Autodesk Inventor part; units mm, degrees
ref_plane "YZ Plane" through (0, 0, 0) normal (1, 0, 0) x (0, 1, 0)
ref_plane "XZ Plane" through (0, 0, 0) normal (0, 1, 0) x (-1, 0, 0)
ref_plane "XY Plane" through (0, 0, 0) normal (0, 0, 1) x (1, 0, 0)
sketch "Schizzo1" plane through (0, 0, 0) normal (0, 1, 0) x (-1, 0, 0)
  circle A0 centre (0, 0) radius 3.25
  circle A1 centre (0, 0) radius 6.5
  dimension "d0" = 6.5
  dimension "d1" = 13
extrude "Estrusione1" add sketch "Schizzo1" along normal blind 15
sketch "Schizzo2" plane through (0, 0, 0) normal (0, -1, 0) x (1, 0, 0)
  line L0 (-13.5, -10) -> (13.5, -10)
  line L1 (13.5, -10) -> (13.5, 10)
  line L2 (13.5, 10) -> (-13.5, 10)
  line L3 (-13.5, 10) -> (-13.5, -10)
  line L4 (-13.5, -10) -> (13.5, 10) construction
  line L5 (13.5, -10) -> (-13.5, 10) construction
  point P0 (0, 0)
  point P1 (0, 0)
  point P2 (0, 0)
  dimension "d4" = 20
  dimension "d5" = 27
extrude "Estrusione2" add sketch "Schizzo2" along normal blind 3
sketch "Schizzo3" plane through (0, -3, 0) normal (0, -1, 0) x (1, 0, 0)
  line L0 (0, 0) -> (-8, 0)
  line L1 (0, 0) -> (8, 0) construction
  line L2 (-8, 0) -> (-8, -5.5)
  line L3 (0, 0) -> (8, 0)
  line L4 (0, 0) -> (8, 0) construction
  line L5 (8, 0) -> (8, -5.5)
  circle A0 centre (0, 0) radius 6.5
  circle A1 centre (0, 0) radius 9.5
  line L6 (-20.3813, -5.5) -> (-15.9716, -5.5)
  line L7 (-20.3813, -5.5) -> (-15.9716, -5.5) construction
  line L8 (-9, -5.5) -> (-7, -5.5)
  line L9 (-9, -5.5) -> (-7, -5.5) construction
  line L10 (-9, -5.5) -> (-7, -5.5) construction
  line L11 (-9, -7.4) -> (-7, -7.4)
  line L12 (-7, -3.6) -> (-9, -3.6)
  arc A2 (-9, -3.6) -> (-9, -7.4) centre (-9, -5.5) ccw
  arc A3 (-7, -7.4) -> (-7, -3.6) centre (-7, -5.5) ccw
  line L13 (7, -5.5) -> (9, -5.5)
  line L14 (7, -5.5) -> (9, -5.5) construction
  line L15 (7, -5.5) -> (9, -5.5) construction
  line L16 (7, -7.4) -> (9, -7.4)
  line L17 (9, -3.6) -> (7, -3.6)
  arc A4 (7, -3.6) -> (7, -7.4) centre (7, -5.5) ccw
  arc A5 (9, -7.4) -> (9, -3.6) centre (9, -5.5) ccw
  point P0 (2.8723, -8)
  point P1 (13.5, -10)
  point P2 (-13.5, -10)
  point P3 (8, -5.5)
  point P4 (0, -10)
  point P5 (0, 10)
  dimension "d21" = 8
  dimension "d22" = 180
  dimension "d23" = 5.5
  dimension "d24" = 90
  dimension "d25" = 8
  dimension "d26" = 0
  dimension "d27" = 5.5
  dimension "d28" = 90
  dimension "d31" = 0
  dimension "d32" = 0
  dimension "d33" = 2
  dimension "d34" = 3.8
  dimension "d35" = 0
  dimension "d36" = 3.8
  dimension "d37" = 2
extrude "Estrusione3" cut sketch "Schizzo3" against normal blind 10 contours L12 A3 A1 L2 | L2 A1 L12 | L17 A1 L5 | L5 A1 A4 L17 | A1 L8 L2 | L2 L8 A1 A3 L11 A2 L12 | A1 L17 A5 L16 A4 L13 L5 | L5 L13 A1
fillet "Raccordo2" radius 2 1 edges at (3.25, 15, 0)
chamfer "Smusso2" distance 3 angle 45 1 edges at (6.5, 0, 0)
fillet "Raccordo3" radius 3 1 edges at (6.5, 3, 0)
sketch "Schizzo4" plane through (0, 0, 0) normal (0, 1, 0) x (1, 0, 0)
  arc A0 (9, 3.6) -> (9, 7.4) centre (9, 5.5) ccw
  arc A1 (7, 7.4) -> (7, 3.6) centre (7, 5.5) ccw
  line L0 (9, 5.5) -> (7, 5.5)
  arc A2 (-9, 7.4) -> (-9, 3.6) centre (-9, 5.5) ccw
  arc A3 (-7, 3.6) -> (-7, 7.4) centre (-7, 5.5) ccw
  line L1 (-9, 5.5) -> (-7, 5.5)
  circle A4 centre (8, 5.5) radius 3
  circle A5 centre (-8, 5.5) radius 3
  line L2 (6.2679, 2.5) -> (4.5359, 5.5)
  line L3 (4.5359, 5.5) -> (6.2679, 8.5)
  line L4 (6.2679, 8.5) -> (9.7321, 8.5)
  line L5 (9.7321, 8.5) -> (11.4641, 5.5)
  line L6 (11.4641, 5.5) -> (9.7321, 2.5)
  line L7 (9.7321, 2.5) -> (6.2679, 2.5)
  line L8 (-6.2679, 8.5) -> (-4.5359, 5.5)
  line L9 (-4.5359, 5.5) -> (-6.2679, 2.5)
  line L10 (-6.2679, 2.5) -> (-9.7321, 2.5)
  line L11 (-9.7321, 2.5) -> (-11.4641, 5.5)
  line L12 (-11.4641, 5.5) -> (-9.7321, 8.5)
  line L13 (-9.7321, 8.5) -> (-6.2679, 8.5)
  point P0 (0, 0)
  point P1 (9.3191, 3.627)
  point P2 (-9.3191, 3.627)
  point P3 (8, 2.5)
  point P4 (-8, 8.5)
  dimension "d45" = 6
  dimension "d46" = 6
extrude "Estrusione6" cut sketch "Schizzo4" along normal blind 6
properties part number "11_Connettore_MPU"
Source: CAD feature listing. Evaluate the final solid. Frame: model axes, mm. A direction names the side the tool comes from. Round coordinates to 2 decimals unless told otherwise and drop trailing zeros. Loops run counter-clockwise (first coordinate to the right, second up) from the corner with the lowest first, then second, coordinate; pieces in that order, holes last. Notation, with made-up numbers: M 72.25,16.25 L 124.25,16.25 A17 ccw 124.25,39.25 Z; hole C -25,-26 d6. An arc over 180 degrees is marked long. Use a Markdown table: item, result. Add a question column.
1. Contact query for flat-ended pins moving along their axis: pin 1 (3 mm diameter, centred on y = 12, z = 0.5, fed in from +X); pin 2 (1.4 mm diameter, centred on x = -8, y = 1, fed in from -Z); pin 3 (8 mm diameter, centred on y = 8, z = 0, fed in from -X). Output: stop coordinate, or through.
2. Set-up query: faces 4 (the flat face through (5, 0.9, -6.3)), 5 (the flat face through (-13.5, -1, 0)), 6 (the flat face through (-4.877, 0.651, -6.091)), 7 (the flat face through (-8, -2, -7.4)), 8 (the cylindrical face through (2.579, 6.409, 1.978)). Return all of +Z, -Z, +X, -X, +Y, -Y with unobstructed straight access to the full face (end or side cutting, diameter ignored); none if empty.
3. Pull-direction query (Z, two-part tool) for faces 1 (the flat face through (7, 1, -2.5)), 2 (the cylindrical face through (-5.1, -1.5, -5.5)), 3 (the conical face through (0.2, 2, 7.5)); classes: +Z half, -Z half, draft (parallel to the pull), parting line (faces both ways), or undercut.
4. Ray query, line 1 along Z through (x, y) = (0, 7.5); line 2 along X through (y, z) = (-1.25, -6.75); line 3 along Y through (x, z) = (9.5, -1.75). Return the intervals inside material, ascending. Write a range as [from, to].
5. Cut plane B-B, the plane x = -10.5. Output: boundary loops of the cut face in (y, z), and give its area (3 significant figures).
6. Cut plane C-C, the plane y = 12.25. Output: boundary loops of the cut face in (x, z), and give its area (3 significant figures).
7. Cut plane D-D, the plane x = 0. Output: boundary loops of the cut face in (y, z), and give its area (3 significant figures).
8. Cut plane A-A, the plane z = 0. Output: boundary loops of the cut face in (x, y), and give its area (3 significant figures).
Solution:
| question | item | result |
|---|---|---|
| 1 | pin 1 | stops at x = 6.5 |
| 1 | pin 2 | stops at z = -2.5 |
| 1 | pin 3 | stops at x = -6.51 |
| 2 | face 4 | +X, +Y |
| 2 | face 5 | +Z, -Z, -X, +Y, -Y |
| 2 | face 6 | -X, +Y |
| 2 | face 7 | +Y, -Y |
| 2 | face 8 | +Y |
| 3 | face 1 | -Z half |
| 3 | face 2 | undercut |
| 3 | face 3 | parting line |
| 4 | line 1 | z = [-6.5, -3.25], [3.25, 6.5] |
| 4 | line 2 | x = [-13.5, -10.43], [-5.57, 5.57], [10.43, 13.5] |
| 4 | line 3 | y = [-3, 0] |
| 5 | outline | M -3,-10 L 0,-10 L 0,-6.67 L -3,-6.67 Z; M -3,-4.33 L 0,-4.33 L 0,10 L -3,10 Z |
| 5 | area | 53.0 mm2 |
| 6 | outline | C 0,0 d13; hole C 0,0 d6.5 |
| 6 | area | 99.5 mm2 |
| 7 | outline | M -3,-10 L 0,-10 L 0,-9.5 L 2.12,-7.38 A3 cw 4.24,-6.5 L 15,-6.5 L 15,-5.25 A2 ccw 13,-3.25 L 0,-3.25 L 0,3.25 L 13,3.25 A2 ccw 15,5.25 L 15,6.5 L 4.24,6.5 A3 cw 2.12,7.38 L 0,9.5 L 0,10 L -3,10 Z |
| 7 | area | 165 mm2 |
| 8 | outline | M -13.5,-3 L 13.5,-3 L 13.5,0 L 9.5,0 L 7.38,2.12 A3 cw 6.5,4.24 L 6.5,15 L 5.25,15 A2 ccw 3.25,13 L 3.25,0 L -3.25,0 L -3.25,13 A2 ccw -5.25,15 L -6.5,15 L -6.5,4.24 A3 cw -7.38,2.12 L -9.5,0 L -13.5,0 Z |
| 8 | area | 186 mm2 |
